Design review of the part built by this model. Coordinates are the model's own, in mm. Face numbers are marked on the shaded views. A direction names the side the tool comes from. Coordinates: 2 decimals unless noted, no trailing zeros. Loops run counter-clockwise (first coordinate to the right, second up) from the corner with the lowest first, then second, coordinate; pieces in that order, holes last. Notation, with made-up numbers: (-21, 11.25) -> (30, 11.25) arc R14 cw to (30, 35.25) -> close; hole circle Ø5 at (72, -37). An arc over 180 degrees is marked (long way). Answer in a Markdown table with one row per item.
```python
from build123d import *

# Parameters (mm, degrees)
SKETCH_1_W          = 10
SKETCH_1_H          = 37
EXTRUDE_1_DEPTH     = 5
CUT_EXTRUDE_1_DEPTH = 3
SKETCH_3_W          = 20
SKETCH_3_H          = 7.5
EXTRUDE_2_DEPTH     = 36
SKETCH_6_W          = 12.25
SKETCH_6_H          = 23
CUT_EXTRUDE_2_DEPTH = 48.027252737
CUT_EXTRUDE_3_REACH = 45.431
SKETCH_7_R          = 1
CUT_EXTRUDE_4_REACH = 52.784
SKETCH_9_R          = 1


with BuildPart() as part:
    # 草图1 → 凸台-拉伸1 (new body)
    with BuildSketch(Plane(origin=(0, 0, 0), x_dir=(1, 0, 0), z_dir=(0, 1, 0))):
        Rectangle(SKETCH_1_W, SKETCH_1_H)
    extrude(amount=-EXTRUDE_1_DEPTH)

    # 草图2 → 切除-拉伸1 (cut)
    with BuildSketch(Plane(origin=(0, 0, 0), x_dir=(1, 0, 0), z_dir=(0, 1, 0))):
        with BuildLine():
            Line((-2.113983221, 14.966101695), (-3.606206671, 0.368644068))
            ThreePointArc((-3.606206671, 0.368644068), (-3.625, 0), (-3.606206671, -0.368644068))
            Line((-3.606206671, -0.368644068), (-2.113983221, -14.966101695))
            ThreePointArc((-2.113983221, -14.966101695), (0, -16.875), (2.113983221, -14.966101695))
            Line((2.113983221, -14.966101695), (3.606206671, -0.368644068))
            ThreePointArc((3.606206671, -0.368644068), (3.625, 0), (3.606206671, 0.368644068))
            Line((3.606206671, 0.368644068), (2.113983221, 14.966101695))
            ThreePointArc((2.113983221, 14.966101695), (0, 16.875), (-2.113983221, 14.966101695))
        make_face()
    extrude(amount=-CUT_EXTRUDE_1_DEPTH, mode=Mode.SUBTRACT)

    # 草图3 → 凸台-拉伸2 (add)
    with BuildSketch(Plane.XZ.offset(5)):
        with Locations((0, -6)):
            Rectangle(SKETCH_3_W, SKETCH_3_H)
    extrude(amount=EXTRUDE_2_DEPTH)

    # 草图6 → 切除-拉伸2 (cut, through all)
    with BuildSketch(Plane.XY.offset(-2.25)):
        with Locations((0, -23)):
            Rectangle(SKETCH_6_W, SKETCH_6_H)
    extrude(amount=-CUT_EXTRUDE_2_DEPTH, mode=Mode.SUBTRACT)

    # 草图7 → 切除-拉伸3 (cut, up to next)
    with BuildSketch(Plane(origin=(0, -3, 0), x_dir=(1, 0, 0), z_dir=(0, 1, 0)), mode=Mode.PRIVATE) as cut_extrude_3_sk1:
        with Locations(Location((0, 12.6, 0), (0, 0, 270))):
            Circle(SKETCH_7_R)
    cut_extrude_3_tool1 = extrude(cut_extrude_3_sk1.sketch, amount=-CUT_EXTRUDE_3_REACH, mode=Mode.PRIVATE) & part.part
    # 草图7 → 切除-拉伸3 (cut, up to next)
    with BuildSketch(Plane(origin=(0, -3, 0), x_dir=(1, 0, 0), z_dir=(0, 1, 0)), mode=Mode.PRIVATE) as cut_extrude_3_sk2:
        with Locations(Location((0, -12.6, 0), (0, 0, 270))):
            Circle(SKETCH_7_R)
    cut_extrude_3_tool2 = extrude(cut_extrude_3_sk2.sketch, amount=-CUT_EXTRUDE_3_REACH, mode=Mode.PRIVATE) & part.part
    add(cut_extrude_3_tool1.solids().sort_by_distance((0, -3, -12.6))[0], mode=Mode.SUBTRACT)
    add(cut_extrude_3_tool2.solids().sort_by_distance((0, -3, 12.6))[0], mode=Mode.SUBTRACT)

    # 草图9 → 切除-拉伸4 (cut, up to next)
    with BuildSketch(Plane(origin=(0, 0, -9.75), x_dir=(-1, 0, 0), z_dir=(0, 0, -1)), mode=Mode.PRIVATE) as cut_extrude_4_sk1:
        with Locations((0, -9.25)):
            Circle(SKETCH_9_R)
    cut_extrude_4_tool1 = extrude(cut_extrude_4_sk1.sketch, amount=-CUT_EXTRUDE_4_REACH, mode=Mode.PRIVATE) & part.part
    # 草图9 → 切除-拉伸4 (cut, up to next)
    with BuildSketch(Plane(origin=(0, 0, -9.75), x_dir=(-1, 0, 0), z_dir=(0, 0, -1)), mode=Mode.PRIVATE) as cut_extrude_4_sk2:
        with Locations((0, -36.75)):
            Circle(SKETCH_9_R)
    cut_extrude_4_tool2 = extrude(cut_extrude_4_sk2.sketch, amount=-CUT_EXTRUDE_4_REACH, mode=Mode.PRIVATE) & part.part
    add(cut_extrude_4_tool1.solids().sort_by_distance((0, -9.25, -9.75))[0], mode=Mode.SUBTRACT)
    add(cut_extrude_4_tool2.solids().sort_by_distance((0, -36.75, -9.75))[0], mode=Mode.SUBTRACT)


solid = part.part
```
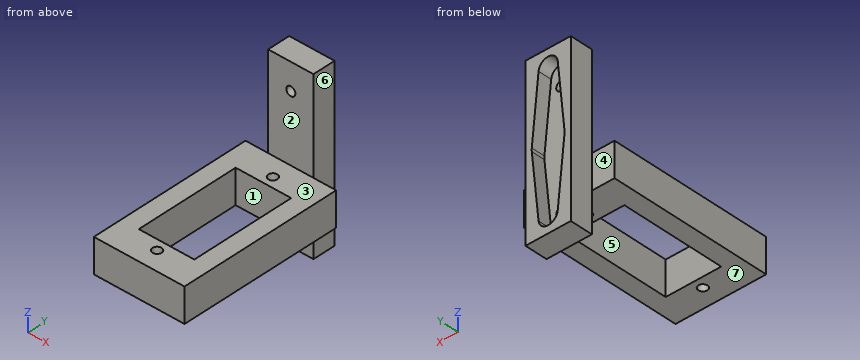
(1) To check wall thickness, follow probe 1 along Y at (x, z) = (0, -5); probe 2 along X at (y, z) = (-4.2, -12.6); probe 3 along Y at (x, z) = (-3.5, -9.5). State the ranges of each line that lie inside material, in increasing order.
Evaluation:
| item | result |
|---|---|
| probe 1 | y = -41 to -37.75, -35.75 to -34.5, -11.5 to -10.25, -8.25 to -3 |
| probe 2 | x = -5 to -1, 1 to 5 |
| probe 3 | y = -41 to -34.5, -11.5 to 0 |
(2) Tool access review of the marked faces 4, 5, 6 and 7: name each direction out of +Z, -Z, +X, -X, +Y, -Y from which nothing blocks a thin tool from reaching the whole face with its end or side.
Evaluation:
| item | result |
|---|---|
| face 4 | +Z, -Z, -X, +Y |
| face 5 | +Z, -Z |
| face 6 | +Z, -Z, +X, +Y |
| face 7 | -Z, +X, -X, -Y |
(3) Take a section at D-D on z = 12.6. Give the boundary of the cut face in (x, y), and give its area (3 significant figures).
Evaluation:
| item | result |
|---|---|
| outline | (-5, -5) -> (-1, -5) -> (-1, -3) -> (-2.36, -3) -> (-2.36, 0) -> (-5, 0) -> close; (1, -5) -> (5, -5) -> (5, 0) -> (2.36, 0) -> (2.36, -3) -> (1, -3) -> close |
| area | 31.9 mm² |
(4) Take a section at B-B on y = -22. Give the boundary of the cut face in (x, z) (3 decimals).
Evaluation:
| item | result |
|---|---|
| outline | (-10, -9.75) -> (-6.125, -9.75) -> (-6.125, -2.25) -> (-10, -2.25) -> close; (6.125, -9.75) -> (10, -9.75) -> (10, -2.25) -> (6.125, -2.25) -> close |
(5) Draft analysis for pull direction Y (two halves, no side actions). For the marked faces 1, 2 and 3, state which applies: pulls with the +Y half, pulls with the -Y half, needs draft (parallel to the pull), parting line crosses it, or undercut.
Evaluation:
| item | result |
|---|---|
| face 1 | undercut |
| face 2 | pulls with the -Y half |
| face 3 | needs draft |
(6) Take a section at A-A on x = 5.5. Give the boundary of the cut face in (y, z), and give its area (3 significant figures).
Evaluation:
| item | result |
|---|---|
| outline | (-41, -9.75) -> (-34.5, -9.75) -> (-34.5, -2.25) -> (-41, -2.25) -> close; (-11.5, -9.75) -> (-5, -9.75) -> (-5, -2.25) -> (-11.5, -2.25) -> close |
| area | 97.5 mm² |
(7) Take a section at C-C on x = 0. Count the separate pieces of the cut face and the enclosed holes in it, and give its area (3 significant figures).
Evaluation:
| item | result |
|---|---|
| separate pieces | 6 |
| enclosed holes | 0 |
| area | 143 mm² |
(8) For pin 1 (2.5 mm diameter, centred on x = 6.5, z = -7.5, fed in from +Y); pin 2 (1.2 mm diameter, centred on x = 0, y = -36.75, fed in from +Z); pin 3 (3 mm diameter, centred on x = 0, y = -9.25, fed in from +Z); pin 4 (6 mm diameter, centred on x = 1.5, z = -2.5, fed in from +Y), all flat-tipped, find the tip position at first contact; note any pin that passes through.
Evaluation:
| item | result |
|---|---|
| pin 1 | stops at y = -5 |
| pin 2 | passes through |
| pin 3 | stops at z = -2.25 |
| pin 4 | stops at y = 0 |
